Work out the finished part from the listing and answer in its coordinate system (mm). Face numbers are marked on the shaded views. A direction names the side the tool comes from. Coordinates: 2 decimals unless noted, no trailing zeros. Order: outer loops, then holes, each group sorted by start corner. A loop starts at its lowest first (then second) coordinate and runs counter-clockwise, first axis right, second up. Notation, with made-up numbers: M -14.5,22 L 36.5,22 A26 ccw 36.5,45 Z; hole C 46.25,-39 d7. An arc over 180 degrees is marked long. Answer in a Markdown table with one row per item. Add a question column.
Item 1: The part is cut by section C-C (y = 6.75). State how many separate pieces and enclosed holes the cut face has, then the cut area to 3 significant figures.
Item 2: Consider line 1 (X direction, y = 14.75, z = 0) (3 decimals); line 2 (X direction, y = 6, z = 23.5); line 3 (Z direction, x = -2.5, y = 18.75). Determine where each line is inside the solid, lowest interval first. Write a range as from..to.
Item 3: The mould has two halves that part along X. Classify the marked faces 1, 2 and 3: released by +X, released by -X, zero draft, split by the parting line, or undercut.
Item 4: Which of the six approach directions +Z, -Z, +X, -X, +Y, -Y give full straight-line access (tool end or side, diameter ignored) to the marked faces 4, 5 and 6?
Item 5: The part is cut by section A-A (x = 0). Write down the section's boundary in (y, z), then the cut area to 3 significant figures.
Item 6: The part is cut by section B-B (z = 15.5). Write down the section's boundary in (x, y), then the cut area to 3 significant figures.
Item 7: The part is cut by section D-D (x = -19). Write down the section's boundary in (y, z).
Item 8: Flat-ended cylindrical pins translate along their axes: pin 1 Ø3 at (x, z) = (25.5, 0) entering from -Y; pin 2 Ø3 at (y, z) = (19.5, -4) entering from +X; pin 3 Ø3 at (y, z) = (8.5, -22.5) entering from -X; pin 4 Ø3 at (y, z) = (19, 9) entering from +X. Find the tip coordinate at first contact, or state that the pin passes through.
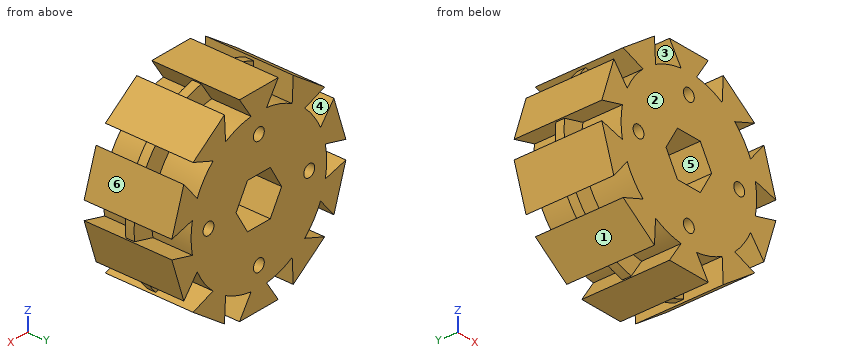
from build123d import *

# Parameters (mm, degrees)
SKETCH1_R           = 22.225
BOSS_EXTRUDE1_DEPTH = 25.4
CUT_EXTRUDE1_DEPTH  = 41.411152545
BOSS_EXTRUDE2_DEPTH = 25.4
CIRPATTERN1_COUNT   = 10
SKETCH5_R           = 27.94
SKETCH5_R_2         = 22.225
BOSS_EXTRUDE3_DEPTH = 1.27
SKETCH6_R           = 1.778
CUT_EXTRUDE2_DEPTH  = 48.329030175


with BuildPart() as part:
    # Sketch1 → Boss-Extrude1 (new body)
    with BuildSketch(Plane(origin=(0, 0, 0), x_dir=(1, 0, 0), z_dir=(0, 1, 0))):
        with Locations(Location((0, 0, 0), (0, 0, 270))):
            Circle(SKETCH1_R)
    extrude(amount=BOSS_EXTRUDE1_DEPTH)

    # Sketch2 → Cut-Extrude1 (cut, through all)
    with BuildSketch(Plane.XZ):
        Polygon((7.478995387, 0), (3.739497694, 6.477), (-3.739497694, 6.477), (-7.478995387, 0), (-3.739497694, -6.477), (3.739497694, -6.477), align=None)
    extrude(amount=-CUT_EXTRUDE1_DEPTH, mode=Mode.SUBTRACT)

    # Sketch3 → Boss-Extrude2 (add)
    with BuildSketch(Plane.XZ):
        with BuildLine():
            Line((-2.54, 22.079380086), (-6.35, 27.94))
            Line((-6.35, 27.94), (6.35, 27.94))
            Line((6.35, 27.94), (2.54, 22.079380086))
            ThreePointArc((2.54, 22.079380086), (0, 22.225), (-2.54, 22.079380086))
        make_face()
    boss_extrude2 = extrude(amount=-BOSS_EXTRUDE2_DEPTH)

    # CirPattern1: Boss-Extrude2 ×10 about axis
    cirpattern1_axis = Axis((0, 0, 0), (0, 1, 0))
    for i in range(1, CIRPATTERN1_COUNT):
        add(boss_extrude2.rotate(cirpattern1_axis, i * 360 / CIRPATTERN1_COUNT))

    # Sketch5 → Boss-Extrude3 (add, symmetric)
    with BuildSketch(Plane(origin=(0, 12.7, 0), x_dir=(1, 0, 0), z_dir=(0, 1, 0))):
        Circle(SKETCH5_R)
        Circle(SKETCH5_R_2, mode=Mode.SUBTRACT)
    extrude(amount=BOSS_EXTRUDE3_DEPTH, both=True)

    # Sketch6 → Cut-Extrude2 (cut, through all)
    with BuildSketch(Plane(origin=(0, 25.4, 0), x_dir=(1, 0, 0), z_dir=(0, 1, 0))):
        with Locations(Location((-16.51, 0, 0), (0, 0, 270))):
            Circle(SKETCH6_R)
        with Locations(Location((0, 16.51, 0), (0, 0, 270))):
            Circle(SKETCH6_R)
        with Locations(Location((16.51, 0, 0), (0, 0, 270))):
            Circle(SKETCH6_R)
        with Locations(Location((0, -16.51, 0), (0, 0, 270))):
            Circle(SKETCH6_R)
    extrude(amount=-CUT_EXTRUDE2_DEPTH, mode=Mode.SUBTRACT)


solid = part.part
Reply:
| question | item | result |
|---|---|---|
| 1 | separate pieces | 1 |
| 1 | enclosed holes | 5 |
| 1 | area | 1,880 mm2 |
| 2 | line 1 | x = -22.225..-18.288, -14.732..-7.479, 7.479..14.732, 18.288..22.225 |
| 2 | line 2 | x = -15.19..-11.14, -3.46..3.46, 11.14..15.19 |
| 2 | line 3 | z = -27.94..-6.48, 6.48..27.94 |
| 3 | face 1 | released by -X |
| 3 | face 2 | zero draft |
| 3 | face 3 | undercut |
| 4 | face 4 | none |
| 4 | face 5 | +Y, -Y |
| 4 | face 6 | +Z, +X, +Y, -Y |
| 5 | outline | M 0,-27.94 L 25.4,-27.94 L 25.4,-18.29 L 0,-18.29 Z; M 0,-14.73 L 25.4,-14.73 L 25.4,-6.48 L 0,-6.48 Z; M 0,6.48 L 25.4,6.48 L 25.4,14.73 L 0,14.73 Z; M 0,18.29 L 25.4,18.29 L 25.4,27.94 L 0,27.94 Z |
| 5 | area | 910 mm2 |
| 6 | outline | M -23.25,11.43 L -15.93,11.43 L -15.93,0 L -1.46,0 L -1.46,25.4 L -15.93,25.4 L -15.93,13.97 L -23.25,13.97 Z; M 1.46,0 L 15.93,0 L 15.93,11.43 L 23.25,11.43 L 23.25,13.97 L 15.93,13.97 L 15.93,25.4 L 1.46,25.4 Z |
| 6 | area | 772 mm2 |
| 7 | outline | M 0,-20.73 L 25.4,-20.73 L 25.4,-17.89 L 13.97,-17.89 L 13.97,-11.53 L 25.4,-11.53 L 25.4,11.53 L 13.97,11.53 L 13.97,17.89 L 25.4,17.89 L 25.4,20.73 L 0,20.73 L 0,17.89 L 11.43,17.89 L 11.43,11.53 L 0,11.53 L 0,-11.53 L 11.43,-11.53 L 11.43,-17.89 L 0,-17.89 Z |
| 8 | pin 1 | stops at y = 11.43 |
| 8 | pin 2 | stops at x = 28.53 |
| 8 | pin 3 | stops at x = -18.63 |
| 8 | pin 4 | stops at x = 26.94 |
